Here's how the part is built. I have some questions about the finished solid (model axes, mm). Face numbers are marked on the shaded views. A direction names the side the tool comes from. Coordinates: 2 decimals unless noted, no trailing zeros. Write each loop counter-clockwise with the first axis right and the second up, starting at its lowest first coordinate (ties: lowest second). Pieces come first, ordered by that corner, then holes.
(1) Please list where these lines run through material, in increasing order: probe 1 along X at (y, z) = (1.1, 13.5); probe 2 along X at (y, z) = (0.2, 13.5); probe 3 along Z at (x, y) = (0, 1.3).
(2) Thinking about a two-plate mould opening in Z: for the marked faces 3, 4 and 5, which applies, released by +Z, released by -Z, zero draft, split by the parting line, or undercut?
(3) For pin 1 Ø3 at (x, z) = (8.5, 1) entering from -Y; pin 2 Ø1.5 at (x, y) = (4.5, 1.5) entering from +Z; pin 3 Ø3 at (x, y) = (-6.5, 2) entering from +Z, each with a flat end and sliding along its axis, tell me the tip position at first contact or that it passes through.
(4) Which directions (+Z, -Z, +X, -X, +Y, -Y) give clear straight access to the entire face, cutting with the end or side of a thin tool? Please do the marked faces 1 and 2.
(5) Imagine slicing it at A-A, the plane z = 19.5. List the corners of the cut face in (x, y) for me.
(6) Imagine slicing it at B-B, the plane y = 1. List the corners of the cut face in (x, z) for me, plus the area to 3 significant figures.
(7) Imagine slicing it at D-D, the plane x = 10.5. State how many separate pieces and enclosed holes the cut face has, plus the area to 3 significant figures.
(8) Imagine slicing it at C-C, the plane x = 0. List the corners of the cut face in (y, z) for me, plus the area to 3 significant figures.
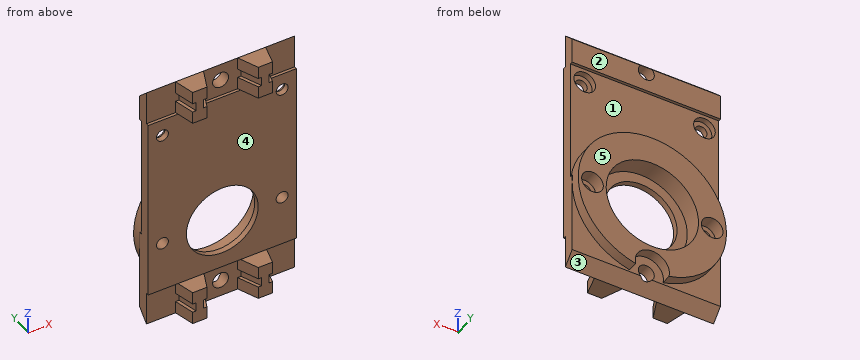
```python
from build123d import *

# Parameters (mm, degrees)
SKETCH_1_W                   = 26
SKETCH_1_H                   = 45
EXTRUDE_1_DEPTH              = 2
EXTRUDE_3_DEPTH              = 6
CUT_EXTRUDE_1_REACH          = 28.561
SKETCH_5_R                   = 1.4
EXTRUDE_4_REACH              = 36.562
SKETCH_6_W                   = 33
SKETCH_6_H                   = 0.5
CUT_EXTRUDE_2_REACH          = 36.562
SKETCH_7_W                   = 22
SKETCH_7_H                   = 0.5
HOLE_WIZARD_M2_1_D           = 2.1
HOLE_WIZARD_M2_1_CBORE_D     = 3.8
HOLE_WIZARD_M2_1_CBORE_DEPTH = 1
CHAMFER_1_SIZE               = 2
EXTRUDE_5_DEPTH              = 2.25
HOLE_WIZARD_M2_2_D           = 2.1
HOLE_WIZARD_M2_2_CBORE_D     = 3.8
HOLE_WIZARD_M2_2_CBORE_DEPTH = 2.25
HOLE_WIZARD_M2_3_D           = 12.6
HOLE_WIZARD_M2_3_CBORE_D     = 16.2
HOLE_WIZARD_M2_3_CBORE_DEPTH = 3.25
CUT_EXTRUDE_3_DEPTH          = 0.8
MIRROR_4_COPY_1_DEPTH        = 0.8


with BuildPart() as part:
    # ｽｹｯﾁ1 → ﾎﾞｽ - 押し出し1 (new body)
    with BuildSketch(Plane(origin=(0, 0, 0), x_dir=(1, 0, 0), z_dir=(0, 1, 0))):
        Rectangle(SKETCH_1_W, SKETCH_1_H)
    extrude(amount=EXTRUDE_1_DEPTH)

    # ｽｹｯﾁ4 → ﾎﾞｽ - 押し出し3 (add)
    with BuildSketch(Plane.XY.offset(22.5)):
        Polygon((-7, -3.5), (-4.5, -3.5), (-3, 0), (-7.9, 0), align=None)
        Polygon((3, 0), (4.5, -3.5), (7, -3.5), (7.9, 0), align=None)
    extrude_3 = extrude(amount=-EXTRUDE_3_DEPTH)

    # ｽｹｯﾁ5 → ｶｯﾄ - 押し出し1 (cut, up to next)
    with BuildSketch(Plane(origin=(0, 2, 0), x_dir=(1, 0, 0), z_dir=(0, 1, 0)), mode=Mode.PRIVATE) as cut_extrude_1_sk1:
        with Locations(Location((0, -19.5, 0), (0, 0, 270))):
            Circle(SKETCH_5_R)
    cut_extrude_1_tool1 = extrude(cut_extrude_1_sk1.sketch, amount=-CUT_EXTRUDE_1_REACH, mode=Mode.PRIVATE) & part.part
    cut_extrude_1 = cut_extrude_1_tool1.solids().sort_by_distance((0, 2, 19.5))[0]
    add(cut_extrude_1, mode=Mode.SUBTRACT)

    # ﾎﾞｽ - 押し出し4: up to this face of the body (flat: up to its plane)
    extrude_4_end = Plane(part.part.faces().sort_by_distance((-13, 1, 0))[0])
    # ｽｹｯﾁ6 → ﾎﾞｽ - 押し出し4 (add, up to the picked face)
    with BuildSketch(Plane(origin=(13, 0, 0), x_dir=(0, 0, -1), z_dir=(1, 0, 0)), mode=Mode.PRIVATE) as extrude_4_sk1:
        with Locations((0, -0.25)):
            Rectangle(SKETCH_6_W, SKETCH_6_H)
    extrude_4_tool1 = split(extrude(extrude_4_sk1.sketch, amount=-EXTRUDE_4_REACH, mode=Mode.PRIVATE), bisect_by=extrude_4_end, keep=Keep.BOTH, mode=Mode.PRIVATE)
    add(extrude_4_tool1.solids().sort_by(Axis((13, -0.25, 0), (-1, 0, 0)))[0])

    # ｽｹｯﾁ7 → ｶｯﾄ - 押し出し2 (cut, up to next)
    with BuildSketch(Plane(origin=(13, 0, 0), x_dir=(0, 0, -1), z_dir=(1, 0, 0)), mode=Mode.PRIVATE) as cut_extrude_2_sk1:
        with Locations((-5, 1.75)):
            Rectangle(SKETCH_7_W, SKETCH_7_H)
    cut_extrude_2_tool1 = extrude(cut_extrude_2_sk1.sketch, amount=-CUT_EXTRUDE_2_REACH, mode=Mode.PRIVATE) & part.part
    add(cut_extrude_2_tool1.solids().sort_by_distance((13, 1.75, 5))[0], mode=Mode.SUBTRACT)

    # M2 丸平ねじ用座ぐり穴1 (through all)
    with Locations(Plane(origin=(0, 1.5, 0), x_dir=(1, 0, 0), z_dir=(0, 1, 0))):
        with Locations((10.5, -13.5)):
            hole_wizard_m2_1 = CounterBoreHole(HOLE_WIZARD_M2_1_D / 2, HOLE_WIZARD_M2_1_CBORE_D / 2, HOLE_WIZARD_M2_1_CBORE_DEPTH)

    # 面取り1
    # the kernel refuses this chamfer: 2 mm, written as the material it takes off along each edge
    with BuildSketch(Plane(origin=(18.143365976, 2, 22.5), x_dir=(0, 0.027495876610586296, -0.9996219169112968), z_dir=(-1, 0, 0))) as chamfer_1_piece_1:
        Polygon((CHAMFER_1_SIZE * 0.999621916911, CHAMFER_1_SIZE * 0.0274958766106), (-CHAMFER_1_SIZE * 0.0274958766106, CHAMFER_1_SIZE * 0.999621916911), (0, 0), align=None)
    extrude(amount=36.286731952, mode=Mode.SUBTRACT)
    with BuildSketch(Plane(origin=(-18.143365976, 2, -22.5), x_dir=(0, -0.9996219169112968, -0.02749587661058563), z_dir=(1, 0, 0))) as chamfer_1_piece_2:
        Polygon((CHAMFER_1_SIZE * 0.999621916911, -CHAMFER_1_SIZE * 0.0274958766106), (-CHAMFER_1_SIZE * 0.0274958766106, -CHAMFER_1_SIZE * 0.999621916911), (0, 0), align=None)
    extrude(amount=36.286731952, mode=Mode.SUBTRACT)

    # ﾐﾗｰ1: ﾎﾞｽ - 押し出し3, ｶｯﾄ - 押し出し1 across plane
    add(extrude_3.mirror(Plane.XY))
    add(cut_extrude_1.mirror(Plane.XY), mode=Mode.SUBTRACT)

    # ｽｹｯﾁ11 → ﾎﾞｽ - 押し出し5 (add)
    with BuildSketch(Plane(origin=(0, 1.5, 0), x_dir=(1, 0, 0), z_dir=(0, 1, 0))):
        with BuildLine():
            ThreePointArc((-2.924988129, 20.166666667), (0, -5.5), (2.924988129, 20.166666667))
            ThreePointArc((2.924988129, 20.166666667), (0, 16.5), (-2.924988129, 20.166666667))
        make_face()
    extrude(amount=EXTRUDE_5_DEPTH)

    # M2 丸平ねじ用座ぐり穴2 (through all)
    with Locations(Plane(origin=(0, 3.75, 0), x_dir=(1, 0, 0), z_dir=(0, 1, 0))):
        with Locations((10.5, 7.5)):
            hole_wizard_m2_2 = CounterBoreHole(HOLE_WIZARD_M2_2_D / 2, HOLE_WIZARD_M2_2_CBORE_D / 2, HOLE_WIZARD_M2_2_CBORE_DEPTH)

    # M2 丸平ねじ用座ぐり穴3 (through all)
    with Locations(Plane(origin=(0, 3.75, 0), x_dir=(1, 0, 0), z_dir=(0, 1, 0))):
        with Locations((0, 7.5)):
            CounterBoreHole(HOLE_WIZARD_M2_3_D / 2, HOLE_WIZARD_M2_3_CBORE_D / 2, HOLE_WIZARD_M2_3_CBORE_DEPTH)

    # ﾐﾗｰ2: M2 丸平ねじ用座ぐり穴1, M2 丸平ねじ用座ぐり穴2 across plane
    add(hole_wizard_m2_1.mirror(Plane(origin=(0, 0, 0), x_dir=(0, 0, 1), z_dir=(1, 0, 0))), mode=Mode.SUBTRACT)
    add(hole_wizard_m2_2.mirror(Plane(origin=(0, 0, 0), x_dir=(0, 0, 1), z_dir=(1, 0, 0))), mode=Mode.SUBTRACT)

    # ｽｹｯﾁ17 → ｶｯﾄ - 押し出し3 (cut, symmetric)
    with BuildSketch(Plane.XY.offset(19.5)):
        Polygon((4.5, -3.5), (3, 0), (3.6, 0), (5.1, -3.5), align=None)
        Polygon((6.4, -3.5), (7, -3.5), (7.9, 0), (7.3, 0), align=None)
    cut_extrude_3 = extrude(amount=CUT_EXTRUDE_3_DEPTH, both=True, mode=Mode.SUBTRACT)

    # ﾐﾗｰ3: ｶｯﾄ - 押し出し3 across plane
    add(cut_extrude_3.mirror(Plane(origin=(0, 0, 0), x_dir=(0, 0, 1), z_dir=(1, 0, 0))), mode=Mode.SUBTRACT)

    # ﾐﾗｰ4: ｶｯﾄ - 押し出し3 across plane
    add(cut_extrude_3.mirror(Plane.XY), mode=Mode.SUBTRACT)

    # ﾐﾗｰ4 copy 1 sketch → ﾐﾗｰ4 copy 1 (cut, symmetric)
    with BuildSketch(Plane(origin=(0, 0, -19.5), x_dir=(-1, 0, 0), z_dir=(0, 0, -1))):
        Polygon((4.5, -3.5), (3, 0), (3.6, 0), (5.1, -3.5), align=None)
        Polygon((6.4, -3.5), (7, -3.5), (7.9, 0), (7.3, 0), align=None)
    extrude(amount=MIRROR_4_COPY_1_DEPTH, both=True, mode=Mode.SUBTRACT)


solid = part.part
```
Recorded:
1. probe 1: x = -13 to -12.4, -8.6 to 8.6, 12.4 to 13
1. probe 2: x = -13 to -11.55, -9.45 to 9.45, 11.55 to 13
1. probe 3: z = -21.2 to -20.9, -18.1 to -15.6, 0.6 to 18.1, 20.9 to 21.2
2. face 3: released by -Z
2. face 4: undercut
2. face 5: zero draft
3. pin 1: stops at y = -0.5
3. pin 2: stops at z = 21.75
3. pin 3: stops at z = 22
4. face 1: +Y
4. face 2: +Z, +X, -X, +Y
5. outline: (-13, 0) - (-7.3, 0) - (-6.4, -3.5) - (-5.1, -3.5) - (-3.6, 0) - (-1.4, 0) - (-1.4, 2) - (-13, 2) - close; (1.4, 0) - (3.6, 0) - (5.1, -3.5) - (6.4, -3.5) - (7.3, 0) - (13, 0) - (13, 2) - (1.4, 2) - close
6. outline: (-13, -21.5) - (13, -21.5) - (13, 21.5) - (-13, 21.5) - close; hole circle Ø3.8 at (-10.5, 13.5); hole circle Ø2.1 at (-10.5, -7.5); hole circle Ø16.2 at (0, -7.5); hole circle Ø2.8 at (0, -19.5); hole circle Ø2.8 at (0, 19.5); hole circle Ø3.8 at (10.5, 13.5); hole circle Ø2.1 at (10.5, -7.5)
6. area: 870 mm2
7. separate pieces: 3
7. enclosed holes: 0
7. area: 103 mm2
8. outline: (-0.5, -16.5) - (0, -16.5) - (0, -18.1) - (2, -18.1) - (2, -16.5) - (3.75, -16.5) - (3.75, -15.6) - (0.5, -15.6) - (0.5, -13.8) - (-0.5, -13.8) - close; (-0.5, -1.2) - (0.5, -1.2) - (0.5, 0.6) - (3.75, 0.6) - (3.75, 5.5) - (1.5, 5.5) - (1.5, 16) - (2, 16) - (2, 18.1) - (0, 18.1) - (0, 16.5) - (-0.5, 16.5) - close; (0, -22.5) - (1.6, -20.9) - (0, -20.9) - close; (0, 20.9) - (1.6, 20.9) - (0, 22.5) - close
8. area: 59.5 mm2
